Model file for the job. Use its own axes, mm. A direction names the side the tool comes from. Give positions to 0.01 mm unless a question says otherwise; leave off trailing zeros. Order: outer loops, then holes, each group sorted by start corner. A loop starts at its lowest first (then second) coordinate and runs counter-clockwise, first axis right, second up. Notation, with made-up numbers: (-14, 36.5) - (43, 36.5) arc R36 cw to (43, 73.5) - close; hole circle Ø3 at (28.5, 8.5). An arc over 180 degrees is marked (long way). Use CSV: the item, a comma, the result in double quotes. Start each with the question number.
(1) Band-saw the part on B-B, the plane x = 28. Give the cut face in (y, z), then the cut area to 3 significant figures.
(2) Tool access for faces 4 (the flat face through (-60, -1, 45)), 5 (the flat face through (-61, -1, 15)), 6 (the flat face through (61, -1, -30)), 7 (the flat face through (61, -1, 15)), 8 (the flat face through (-41.43, -1.44, 43.495)): list every direction of +Z, -Z, +X, -X, +Y, -Y with a clear straight run to the whole face (end or side of a thin tool).
(3) Probe L1, parallel to Z at x = 0.5, y = -1; L2, parallel to Z at x = -42.5, y = -2.1; L3, parallel to X at y = -0.85, z = -46. List the from-to ranges inside material, lowest first.
(4) Drop flat-ended pins along their axis: pin 1 Ø1.5 at (y, z) = (-2, -61) entering from +X; pin 2 Ø1.5 at (y, z) = (-1.5, 61.5) entering from -X; pin 3 Ø1.5 at (x, y) = (-61.5, -2) entering from +Z. Give the stop position or say it passes through.
(5) Band-saw the part on A-A, the plane z = 50. Give the cut face in (x, y).
(6) Pull direction X, two halves, no side cores. Call faces 1 (the cylindrical face through (0.584, -1.44, -54.997)), 2 (the flat face through (-61, -1, -30)), 3 (the flat face through (60, -1, 0)): +X half, -X half, draft (parallel to the pull), parting line (faces both ways), or undercut.
from build123d import *

# Parameters (mm, degrees)
F2_DEPTH = 2.92


with BuildPart() as f2:
    # F1 (on Front) → F2 (new body)
    with BuildSketch(Plane.XZ):
        Polygon((-7.5, 60), (-60, 60), (-60, 30), (-62.92, 30), (-62.92, 15), (-60, 15), (-60, 0), (-60, -15), (-62.92, -15), (-62.92, -30), (-60, -30), (-60, -60), (-7.5, -60), (-7.5, -62.92), (7.5, -62.92), (7.5, -60), (60, -60), (60, -30), (62.92, -30), (62.92, -15), (60, -15), (60, 0), (60, 15), (62.92, 15), (62.92, 30), (60, 30), (60, 60), (7.5, 60), (7.5, 62.92), (-7.5, 62.92), align=None)
        with BuildLine():
            ThreePointArc((-39.9095440073, -37.8447922062), (-55, 0), (-39.9095440073, 37.8447922062))
            Line((-39.9095440073, 37.8447922062), (-46.9806118191, 44.9158600181))
            Line((-46.9806118191, 44.9158600181), (-44.9158600181, 46.9806118191))
            Line((-44.9158600181, 46.9806118191), (-37.8447922062, 39.9095440073))
            ThreePointArc((-37.8447922062, 39.9095440073), (0, 55), (37.8447922062, 39.9095440073))
            Line((37.8447922062, 39.9095440073), (44.9158600181, 46.9806118191))
            Line((44.9158600181, 46.9806118191), (46.9806118191, 44.9158600181))
            Line((46.9806118191, 44.9158600181), (39.9095440073, 37.8447922062))
            ThreePointArc((39.9095440073, 37.8447922062), (55, 0), (39.9095440073, -37.8447922062))
            Line((39.9095440073, -37.8447922062), (46.9806118191, -44.9158600181))
            Line((46.9806118191, -44.9158600181), (44.9158600181, -46.9806118191))
            Line((44.9158600181, -46.9806118191), (37.8447922062, -39.9095440073))
            ThreePointArc((37.8447922062, -39.9095440073), (0, -55), (-37.8447922062, -39.9095440073))
            Line((-37.8447922062, -39.9095440073), (-44.9158600181, -46.9806118191))
            Line((-44.9158600181, -46.9806118191), (-46.9806118191, -44.9158600181))
            Line((-46.9806118191, -44.9158600181), (-39.9095440073, -37.8447922062))
        make_face(mode=Mode.SUBTRACT)
    extrude(amount=F2_DEPTH)


solid = f2.part
Answer block:
1,outline,"(-2.92, -60) - (0, -60) - (0, -47.34) - (-2.92, -47.34) - close; (-2.92, 47.34) - (0, 47.34) - (0, 60) - (-2.92, 60) - close"
1,area,"73.9 mm2"
2,face 4,"+Z, -X, +Y, -Y"
2,face 5,"-X, +Y, -Y"
2,face 6,"-Z, +X, +Y, -Y"
2,face 7,"+X, +Y, -Y"
2,face 8,"+Y, -Y"
3,L1,"z = -62.92 to -55, 55 to 62.92"
3,L2,"z = -60 to -44.56, -40.44 to -34.91, 34.91 to 40.44, 44.56 to 60"
3,L3,"x = -60 to -45.9, -43.94 to -30.15, 30.15 to 43.94, 45.9 to 60"
4,pin 1,"stops at x = 7.5"
4,pin 2,"stops at x = -7.5"
4,pin 3,"stops at z = 30"
5,outline,"(-60, -2.92) - (-22.91, -2.92) - (-22.91, 0) - (-60, 0) - close; (22.91, -2.92) - (60, -2.92) - (60, 0) - (22.91, 0) - close"
6,face 1,"undercut"
6,face 2,"draft"
6,face 3,"+X half"
